Check sheet for the modelled part. Datum: model origin and axes. Units: mm. A direction names the side the tool comes from. Round coordinates to 2 decimals unless told otherwise and drop trailing zeros. Loops run counter-clockwise (first coordinate to the right, second up) from the corner with the lowest first, then second, coordinate; pieces in that order, holes last. Notation, with made-up numbers: (46, 70) - (97, 70) arc R28 ccw to (97, 99) - close; hole circle Ø6 at (-30.5, -20.75). An arc over 180 degrees is marked (long way). Put each result on its own line as item: value.
```python
from build123d import *

# Parameters (mm, degrees)
BOSS_EXTRUDE1_DEPTH                                 = 4
CSK_FOR_M3_COUNTERSUNK_FLAT_HEAD_SCREW1_D           = 3.4
CSK_FOR_M3_COUNTERSUNK_FLAT_HEAD_SCREW1_CSINK_D     = 6.3
CSK_FOR_M3_COUNTERSUNK_FLAT_HEAD_SCREW1_CSINK_ANGLE = 90
CSK_FOR_M3_COUNTERSUNK_FLAT_HEAD_SCREW2_D           = 3.4
CSK_FOR_M3_COUNTERSUNK_FLAT_HEAD_SCREW2_CSINK_D     = 6.3
CSK_FOR_M3_COUNTERSUNK_FLAT_HEAD_SCREW2_CSINK_ANGLE = 90
CUT_EXTRUDE1_DEPTH                                  = 4


with BuildPart() as part:
    # Sketch1 → Boss-Extrude1 (new body)
    with BuildSketch(Plane(origin=(0, 0, 0), x_dir=(1, 0, 0), z_dir=(0, 1, 0))):
        with BuildLine():
            Line((-15, -20), (15, -20))
            ThreePointArc((15, -20), (18.535533906, -18.535533906), (20, -15))
            Line((20, -15), (20, 15))
            ThreePointArc((20, 15), (18.535533906, 18.535533906), (15, 20))
            Line((15, 20), (-15, 20))
            ThreePointArc((-15, 20), (-18.535533906, 18.535533906), (-20, 15))
            Line((-20, 15), (-20, -15))
            ThreePointArc((-20, -15), (-18.535533906, -18.535533906), (-15, -20))
        make_face()
    extrude(amount=BOSS_EXTRUDE1_DEPTH)

    # CSK for M3 Countersunk Flat Head Screw1 (through all)
    with Locations(Plane(origin=(-14, 4, -14), x_dir=(0, 0, 1), z_dir=(0, 1, 0))):
        with Locations((0, 0), (0, 28), (28, 28), (28, 0)):
            CounterSinkHole(CSK_FOR_M3_COUNTERSUNK_FLAT_HEAD_SCREW1_D / 2, CSK_FOR_M3_COUNTERSUNK_FLAT_HEAD_SCREW1_CSINK_D / 2, counter_sink_angle=CSK_FOR_M3_COUNTERSUNK_FLAT_HEAD_SCREW1_CSINK_ANGLE)

    # CSK for M3 Countersunk Flat Head Screw2 (through all)
    with Locations(Plane(origin=(0, 0, 0), x_dir=(-1, 0, 0), z_dir=(0, -1, 0))):
        with Locations((3.5, 0.2), (3.5, -6.8)):
            CounterSinkHole(CSK_FOR_M3_COUNTERSUNK_FLAT_HEAD_SCREW2_D / 2, CSK_FOR_M3_COUNTERSUNK_FLAT_HEAD_SCREW2_CSINK_D / 2, counter_sink_angle=CSK_FOR_M3_COUNTERSUNK_FLAT_HEAD_SCREW2_CSINK_ANGLE)

    # Sketch7 → Cut-Extrude1 (cut)
    with BuildSketch(Plane(origin=(0, 4, 0), x_dir=(1, 0, 0), z_dir=(0, 1, 0))):
        Polygon((-12.263344174, 7.136676397), (-11.15360872, 7.136676397), (-11.15360872, 4.150967788), (-8.022255789, 4.150967788), (-8.022255789, 3.041232335), (-11.15360872, 3.041232335), (-11.15360872, 0.055523726), (-12.263344174, 0.055523726), (-12.263344174, 3.041232335), (-15.370423051, 3.041232335), (-15.370423051, 4.150967788), (-12.263344174, 4.150967788), align=None)
        with BuildLine():
            add(Edge.make_bspline(
                [(-15.043692162, -4.829120306), (-14.880436161, -4.763861041), (-14.5584639, -4.635157209), (-14.077627456, -4.457919156), (-13.607003536, -4.298363006), (-13.296000815, -4.200734384), (-13.143053989, -4.152721981)],
                knots=[0, 0, 0, 0, 0.000527431, 0.001040195, 0.001537166, 0.002018074, 0.002018074, 0.002018074, 0.002018074], degree=3))
            Line((-13.143053989, -4.152721981), (-13.142217189, -4.129946622))
            add(Edge.make_bspline(
                [(-13.142217189, -4.129946622), (-13.300142366, -4.076064923), (-13.613682824, -3.969089626), (-14.081290903, -3.798233499), (-14.553659216, -3.619087412), (-14.870442844, -3.493499611), (-15.032410797, -3.429287962)],
                knots=[0, 0, 0, 0, 0.000500579, 0.000993836, 0.001493443, 0.002016132, 0.002016132, 0.002016132, 0.002016132], degree=3))
            Line((-15.032410797, -3.429287962), (-17.320356965, -2.510346296))
            Line((-17.320356965, -2.510346296), (-17.320356965, -0.507736863))
            Line((-17.320356965, -0.507736863), (-11.797862272, -3.15360872))
            Line((-11.797862272, -3.15360872), (-8.007023631, -3.15360872))
            Line((-8.007023631, -3.15360872), (-8.007023631, -4.937612774))
            Line((-8.007023631, -4.937612774), (-11.858418799, -4.937612774))
            Line((-11.858418799, -4.937612774), (-17.320356965, -7.7048549))
            Line((-17.320356965, -7.7048549), (-17.320356965, -5.726519521))
            Line((-17.320356965, -5.726519521), (-15.043692162, -4.829120306))
        make_face()
    extrude(amount=-CUT_EXTRUDE1_DEPTH, mode=Mode.SUBTRACT)


solid = part.part
```
Item 1: Section check B-B on x = 14. Enter the section's corners in (y, z), then the cut area to 3 significant figures.
Filled sheet:
outline: (0, -20) - (4, -20) - (4, -17.15) - (2.55, -15.7) - (0, -15.7) - close; (0, -12.3) - (2.55, -12.3) - (4, -10.85) - (4, 10.85) - (2.55, 12.3) - (0, 12.3) - close; (0, 15.7) - (2.55, 15.7) - (4, 17.15) - (4, 20) - (0, 20) - close
area: 129 mm²
Item 2: Section check D-D on x = -14. Count the separate pieces of the cut face and the enclosed holes in it, then the cut area to 3 significant figures.
Filled sheet:
separate pieces: 6
enclosed holes: 0
area: 111 mm²
Item 3: Tool access check on faces 1 (the flat face through (-16.198, 2.028, 5.284)), 2 (the flat face through (0, 4, 0)). Record the directions out of +Z, -Z, +X, -X, +Y, -Y that give a thin tool (end or side, any length) a straight path to the whole face; none if there is none.
Filled sheet:
face 1: +Y, -Y
face 2: +Z, -Z, +X, -X, +Y
Item 4: Go/stop test with a flat-tipped pin: pin 1 (4 mm diameter, centred on x = -14, z = -14, fed in from +Y). Record where the tip stops, or that it passes through.
Filled sheet:
pin 1: y = 2.85
Item 5: Section check C-C on z = -5. Enter the section's corners in (x, y).
Filled sheet:
outline: (-20, 0) - (-12.26, 0) - (-12.26, 4) - (-20, 4) - close; (-11.15, 0) - (20, 0) - (20, 4) - (-11.15, 4) - close
Item 6: Section check A-A on z = 14. Enter the section's corners in (x, y), then the cut area to 3 significant figures.
Filled sheet:
outline: (-20, 0) - (-15.7, 0) - (-15.7, 2.55) - (-17.15, 4) - (-20, 4) - close; (-12.3, 0) - (12.3, 0) - (12.3, 2.55) - (10.85, 4) - (-10.85, 4) - (-12.3, 2.55) - close; (15.7, 0) - (20, 0) - (20, 4) - (17.15, 4) - (15.7, 2.55) - close
area: 129 mm²
Item 7: Thickness scan on line 1 (Z direction, x = 14, y = 1.25); line 2 (Z direction, x = -11, y = 1.2). Record the ranges inside material, lowest first. Write a range as from..to.
Filled sheet:
line 1: -20..-15.7, -12.3..12.3, 15.7..20
line 2: -20..-4.15, -3.04..3.15, 4.94..20
Item 8: Release check for a two-part mould opening along Z. For faces 3 (the flat face through (20, 2, 0)), 4 (the flat face through (-17.32, 2, 2)), 5 (the cylindrical face through (-13.49, 1.26, 12.38)), 6 (the flat face through (0, 2, 20)) record: +Z half, -Z half, draft (parallel to the pull), parting line (faces both ways), or undercut.
Filled sheet:
face 3: draft
face 4: undercut
face 5: undercut
face 6: +Z half
